For this review, take the finished solid that the model builds, in its own axes (mm). A direction names the side the tool comes from. Round coordinates to 2 decimals unless told otherwise and drop trailing zeros. Write each loop counter-clockwise with the first axis right and the second up, starting at its lowest first coordinate (ties: lowest second). Pieces come first, ordered by that corner, then holes. Notation, with made-up numbers: (53.25, 27.25) -> (67.25, 27.25) arc R5 ccw to (67.25, 32.25) -> close; hole circle Ø1 at (79, 50.5). An arc over 180 degrees is marked (long way). Write each question's results on one line, items separated by ' | '. Start each with the question number.
Item 1: The part is to be moulded in two halves that separate along Y. For faces 1 (the cylindrical face through (-2.58, 2.41, -4.05)), 2 (the cylindrical face through (-4.032, 0.913, -6.324)), 3 (the flat face through (3, 7.8, -4)), 4 (the flat face through (0, 18, 5)), say which applies: +Y half, -Y half, draft (parallel to the pull), parting line (faces both ways), or undercut.
Item 2: Add section B-B (y = -22). State the section outline as (x, z) points.
Item 3: Clearance check with flat-ended pins moving along their axes: pin 1 (12 mm diameter, centred on x = -8.5, y = 9.5, fed in from +Z); pin 2 (10 mm diameter, centred on x = 0, y = -13.5, fed in from +Z); pin 3 (10 mm diameter, centred on x = 6, y = -21.5, fed in from +Z). State where each tip first meets the part, or that it passes through.
Item 4: To check wall thickness, follow line 1 along X through (y, z) = (16, -2.25); line 2 along Y through (x, z) = (4, 1.5); line 3 along Y through (x, z) = (-9, -7.5). State the ranges of each line that lie inside material, in increasing order.
Item 5: Add section A-A (y = 7). State the section outline as (x, z) points, plus the area to 3 significant figures.
Item 6: Tool access review of faces 5 (the flat face through (0, -36, 0)), 6 (the flat face through (0, 1.8, 5)): name each direction out of +Z, -Z, +X, -X, +Y, -Y from which nothing blocks a thin tool from reaching the whole face with its end or side.
from build123d import *

# Parameters (mm, degrees)
FILLET1_R     = 2
SCALE_1_SCALE = 0.6


with BuildPart() as part:
    # Sketch1 → Revolve1 (revolve)
    with BuildSketch(Plane.XY, mode=Mode.PRIVATE) as revolve1_sk:
        with BuildLine():
            Line((0, -60), (20, -60))
            Line((20, -60), (20, -55))
            ThreePointArc((20, -55), (11.03487717, -28.14693589), (8, 0))
            Line((8, 0), (12.5, 0))
            Line((12.5, 0), (12.5, 3))
            Line((12.5, 3), (8, 3))
            Line((8, 3), (8, 5))
            ThreePointArc((8, 5), (6.5, 6.5), (8, 8))
            Line((8, 8), (8, 10))
            Line((8, 10), (10, 10))
            Line((10, 10), (10, 13))
            Line((10, 13), (8, 13))
            ThreePointArc((8, 13), (8.976394405, 21.837130893), (12.5, 30))
            Line((12.5, 30), (8, 30))
            ThreePointArc((8, 30), (6.617187865, 34.495867521), (2.946793809, 37.4375))
            ThreePointArc((2.946793809, 37.4375), (2.311655251, 39.912132318), (0, 41))
            Line((0, 41), (0, -60))
        make_face()
    revolve(revolve1_sk.sketch.rotate(Axis((0, 50, 0), (0, -1, 0)), 180), axis=Axis((0, 50, 0), (0, -1, 0)))

    # Fillet1
    fillet1_edges = [part.edges().sort_by_distance(p)[0] for p in [
        (8, 0, 0),
    ]]
    fillet(fillet1_edges, radius=FILLET1_R)


with BuildPart() as part_1:
    # 缩放比例1: scaled about (0, 0, 0)
    add(part.part.scale(SCALE_1_SCALE))


solid = part_1.part
Responses:
1) face 1: undercut | face 2: draft | face 3: undercut | face 4: +Y half
2) outline: circle Ø15.83 at (0, 0)
3) pin 1: stops at z = 5.33 | pin 2: stops at z = 6.99 | pin 3: stops at z = 8.52
4) line 1: x = -6.02 to 6.02 | line 2: y = -36 to 3.17, 4.63 to 20.19 | line 3: y = -36 to -32.37
5) outline: circle Ø12 at (0, 0) | area: 113 mm^2
6) face 5: +Z, -Z, +X, -X, -Y | face 6: none
